Design review of the part built by this model. Coordinates are the model's own, in mm. A direction names the side the tool comes from. Give positions to 0.01 mm unless a question says otherwise; leave off trailing zeros. Order: outer loops, then holes, each group sorted by start corner. A loop starts at its lowest first (then second) coordinate and runs counter-clockwise, first axis right, second up. Notation, with made-up numbers: M 52,26.25 L 101,26.25 A7 cw 101,37.25 Z; hole C -17.75,50 d11. An arc over 180 degrees is marked long. Answer as a JSON object with one key per item and string values.
from build123d import *

# Parameters (mm, degrees)
SKETCH1_R               = 9.525
BOSS_EXTRUDE1_DEPTH     = 6.35
SKETCH2_R               = 3.175
BOSS_EXTRUDE2_DEPTH     = 4.7752
CUT_EXTRUDE1_DEPTH      = 23.064312023
CUT_EXTRUDE1_DEPTH_BACK = 23.064312023
SKETCH3_W               = 7.260653016
SKETCH3_H               = 19.707486758
SKETCH3_W_2             = 5.945134003
SKETCH3_H_2             = 19.682188315
CUT_EXTRUDE2_DEPTH      = 23.069793838
CUT_EXTRUDE2_DEPTH_BACK = 23.069793838
SKETCH4_R               = 3.175


with BuildPart() as part:
    # Sketch1 → Boss-Extrude1 (new, symmetric)
    with BuildSketch(Plane(origin=(0, 0, 0), x_dir=(0, 0, -1), z_dir=(1, 0, 0))):
        Circle(SKETCH1_R)
    extrude(amount=BOSS_EXTRUDE1_DEPTH, both=True)

    # Sketch2 → Boss-Extrude2 (add)
    with BuildSketch(Plane(origin=(6.35, 0, 0), x_dir=(0, 0, -1), z_dir=(1, 0, 0))):
        Circle(SKETCH2_R)
    boss_extrude2 = extrude(amount=BOSS_EXTRUDE2_DEPTH)

    # Mirror1: Boss-Extrude2 across plane
    add(boss_extrude2.mirror(Plane(origin=(0, 0, 0), x_dir=(0, 0, 1), z_dir=(1, 0, 0))))

    # Sketch3 → Cut-Extrude1 (cut, two sides: drawn at the far end of the back side and taken through both)
    with BuildSketch(Plane(origin=(6.35, 0, 0), x_dir=(0, 0, -1), z_dir=(1, 0, 0)).offset(-CUT_EXTRUDE1_DEPTH_BACK)):
        with Locations((-11.885326508, -0.354178196)):
            Rectangle(SKETCH3_W, SKETCH3_H)
        with Locations((11.227567002, -0.695707171)):
            Rectangle(SKETCH3_W_2, SKETCH3_H_2)
    extrude(amount=CUT_EXTRUDE1_DEPTH + CUT_EXTRUDE1_DEPTH_BACK, mode=Mode.SUBTRACT)

    # Sketch4 → Cut-Extrude2 (cut, two sides: drawn at the far end of the back side and taken through both)
    with BuildSketch(Plane.XY.offset(8.255).offset(-CUT_EXTRUDE2_DEPTH_BACK)):
        Circle(SKETCH4_R)
    extrude(amount=CUT_EXTRUDE2_DEPTH + CUT_EXTRUDE2_DEPTH_BACK, mode=Mode.SUBTRACT)


solid = part.part
(1) We need section D-D (x = 2.5). Write out the cut boundary in (y, z) (3 decimals).
Checked values:
{"outline": "M -4.752,-8.255 L -1.957,-8.255 L -1.957,8.255 L -4.752,8.255 A9.525 ccw Z; M 1.957,-8.255 L 4.752,-8.255 A9.525 ccw 4.752,8.255 L 1.957,8.255 Z"}
(2) Draft analysis for pull direction Y (two halves, no side actions). For faces 3 (the cylindrical face through (-0.69, -3.1, -0.12)), 4 (the cylindrical face through (-8.7, -3.1, 0.69)), 5 (the flat face through (-6.35, 0, -4)), 6 (the cylindrical face through (0.089, 9.524, -0.14)), state which applies: +Y half, -Y half, draft (parallel to the pull), parting line (faces both ways), or undercut.
Checked values:
{"face 3": "undercut", "face 4": "parting line", "face 5": "draft", "face 6": "+Y half"}
(3) We need section C-C (z = 0). Write out the cut boundary in (x, y) (3 decimals).
Checked values:
{"outline": "M -11.125,-3.175 L -6.35,-3.175 L -6.35,-9.525 L 6.35,-9.525 L 6.35,-3.175 L 11.125,-3.175 L 11.125,3.175 L 6.35,3.175 L 6.35,9.525 L -6.35,9.525 L -6.35,3.175 L -11.125,3.175 Z; hole C 0,0 d6.35"}
(4) We need section A-A (x = 0). Write out the cut boundary in (y, z) (3 decimals).
Checked values:
{"outline": "M -4.752,-8.255 L -3.175,-8.255 L -3.175,8.255 L -4.752,8.255 A9.525 ccw Z; M 3.175,-8.255 L 4.752,-8.255 A9.525 ccw 4.752,8.255 L 3.175,8.255 Z"}
(5) To check wall thickness, follow L1, parallel to X at y = 0, z = -1.25 (3 decimals); L2, parallel to X at y = 0, z = -4.25 (3 decimals); L3, parallel to Y at x = 0, z = 5.5 (3 decimals). State the ranges of each line that lie inside material, in increasing order. Write a range as from..to.
Checked values:
{"L1": "x = -11.125..-3.175, 3.175..11.125", "L2": "x = -6.35..-3.175, 3.175..6.35", "L3": "y = -7.777..-3.175, 3.175..7.777"}
(6) Tool access review of faces 1 (the flat face through (11.125, 0, 0)), 2 (the flat face through (6.35, 0, -4)): name each direction out of +Z, -Z, +X, -X, +Y, -Y from which nothing blocks a thin tool from reaching the whole face with its end or side.
Checked values:
{"face 1": "+Z, -Z, +X, +Y, -Y", "face 2": "+X"}
(7) We need section B-B (y = 0). Write out the cut boundary in (x, z) (3 decimals), plus the area to 3 significant figures.
Checked values:
{"outline": "M -11.125,-3.175 L -6.35,-3.175 L -6.35,-8.255 L -3.175,-8.255 L -3.175,8.255 L -6.35,8.255 L -6.35,3.175 L -11.125,3.175 Z; M 3.175,-8.255 L 6.35,-8.255 L 6.35,-3.175 L 11.125,-3.175 L 11.125,3.175 L 6.35,3.175 L 6.35,8.255 L 3.175,8.255 Z", "area": "165 mm^2"}
(8) Insertion check: pin 1 (2 mm diameter, centred on y = -4.5, z = -4.5, fed in from +X); pin 2 (6 mm diameter, centred on x = 2, z = 6.5, fed in from +Y); pin 3 (2 mm diameter, centred on x = 7.5, z = 2, fed in from -Y). Each pin has a flat end and moves straight along its axis. Give the tip position at first contact, or say it passes through.
Checked values:
{"pin 1": "stops at x = 6.35", "pin 2": "stops at y = 8.86", "pin 3": "stops at y = -3.01"}
